For this review, take the finished solid that the model builds, in its own axes (mm). A direction names the side the tool comes from. Give positions to 0.01 mm unless a question says otherwise; leave off trailing zeros. Use a Markdown table: item, result. Add a question column.
1) Machinability: for faces 1 (the face through (0, 22, -5)), 2 (the face through (-22, 0, 5)), 3 (the face through (0, -22, -5)), 4 (the face through (-22.3, 0.1, -6.5)), which of the approach directions +Z, -Z, +X, -X, +Y, -Y give a long, thin tool a straight path to every point of the face, cutting with its end or side? Answer none if there is none.
2) Mouldability with a two-part tool opening along Z and no side actions: class faces 5 (the face through (-22.3, 0.1, 6.5)), 6 (the face through (-25, 0, 0)), 7 (the face through (0, 0, 50)) as released by +Z, released by -Z, zero draft, split by the parting line, or undercut.
3) Wall thickness on L1, parallel to Z at x = 18.5, y = 22.5; L2, parallel to X at y = 12.5, z = 4: over which ranges is each line inside the solid? List them lowest first.
4) Clearance check with flat-ended pins moving along their axes: P1, Ø2.5, axis at x = -7, z = -5, coming from the -Y side; P2, Ø1.5, axis at y = 9, z = -4.5, coming from the +X side; P3, Ø0.9, axis at y = -2.5, z = -5, coming from the -X side. State where each tip first meets the part, or that it passes through.
```python
from build123d import *

# Parameters (mm, degrees)
SKETCH1_W           = 100
SKETCH1_H           = 50
BOSS_EXTRUDE1_DEPTH = 25
SKETCH2_W           = 50
SKETCH2_H           = 50
SKETCH2_W_2         = 44
SKETCH2_H_2         = 44
CUT_EXTRUDE1_DEPTH  = 1.5


with BuildPart() as part:
    # Sketch1 → Boss-Extrude1 (new, symmetric)
    with BuildSketch(Plane(origin=(0, 0, 0), x_dir=(0, 0, -1), z_dir=(1, 0, 0))):
        Rectangle(SKETCH1_W, SKETCH1_H)
    extrude(amount=BOSS_EXTRUDE1_DEPTH, both=True)

    # Sketch2 → Cut-Extrude1 (cut, symmetric)
    with BuildSketch(Plane.XY.offset(5)):
        Rectangle(SKETCH2_W, SKETCH2_H)
        Rectangle(SKETCH2_W_2, SKETCH2_H_2, mode=Mode.SUBTRACT)
    cut_extrude1 = extrude(amount=CUT_EXTRUDE1_DEPTH, both=True, mode=Mode.SUBTRACT)

    # Mirror1: Cut-Extrude1 across plane
    add(cut_extrude1.mirror(Plane.XY), mode=Mode.SUBTRACT)


solid = part.part
```
Checked values:
| question | item | result |
|---|---|---|
| 1 | face 1 | +X, -X, +Y |
| 1 | face 2 | -X, +Y, -Y |
| 1 | face 3 | +X, -X, -Y |
| 1 | face 4 | none |
| 2 | face 5 | undercut |
| 2 | face 6 | zero draft |
| 2 | face 7 | released by +Z |
| 3 | L1 | -50 to -6.5, -3.5 to 3.5, 6.5 to 50 |
| 3 | L2 | -22 to 22 |
| 4 | P1 | y = -22 |
| 4 | P2 | x = 22 |
| 4 | P3 | x = -22 |
